Autodesk Inventor part; units mm, degrees
ref_plane "YZ Plane" through (0, 0, 0) normal (1, 0, 0) x (0, 1, 0)
ref_plane "XZ Plane" through (0, 0, 0) normal (0, 1, 0) x (-1, 0, 0)
ref_plane "XY Plane" through (0, 0, 0) normal (0, 0, 1) x (1, 0, 0)
sketch "Sketch1" plane through (0, 0, 0) normal (0, 1, 0) x (-1, 0, 0)
  point P0 (0, 0)
sketch "Sketch2" plane through (0, 0, 0) normal (0, 1, 0) x (-1, 0, 0)
  line L0 (0, 0) -> (35, 0)
  line L1 (35, 0) -> (35, 25)
  line L2 (35, 25) -> (0, 25)
  line L3 (0, 25) -> (0, 0)
  dimension "d0" = 35
  dimension "d1" = 25
extrude "Extrusion1" add sketch "Sketch2" along normal blind 8
sketch "Sketch3" plane through (0, 8, 0) normal (0, 1, 0) x (1, 0, 0)
  line L0 (-28.1608, -22.5) -> (-6.6608, -22.5)
  line L1 (-6.6608, -22.5) -> (-6.6608, -6)
  line L2 (-6.6608, -6) -> (-28.1608, -6)
  line L3 (-28.1608, -6) -> (-28.1608, -22.5)
  dimension "d4" = 21.5
  dimension "d5" = 16.5
extrude "Extrusion2" cut sketch "Sketch3" against normal blind 4
sketch "Sketch4" plane through (-6.6608, 8, 22.5) normal (0, 0, -1) x (-1, 0, 0)
  point P0 (-6.6608, -8)
sketch "Sketch5" plane through (-28.1608, 8, 6) normal (0, 0, 1) x (1, 0, 0)
  line L0 (0, -4) -> (21.5, -4)
  line L1 (21.5, -4) -> (21.5, 0)
  line L2 (21.5, 0) -> (0, 0)
  line L3 (0, 0) -> (0, -4)
  point P0 (28.1608, -8)
sketch "Sketch12" plane through (0, 8, 0) normal (0, 1, 0) x (1, 0, 0)
  line L0 (-28.1608, -6) -> (-6.6608, -6)
  line L1 (0, 0) -> (-35, 0)
  line L2 (-15, -6) -> (-20, -6)
  line L3 (-20, -6) -> (-20, 0)
  line L4 (-20, 0) -> (-15, 0)
  line L5 (-15, 0) -> (-15, -6)
  dimension "d27" = 5
extrude "Extrusion9" cut sketch "Sketch12" against normal blind 2.5
fillet "Fillet1" radius 2 1 edges at (-35, 4, 0)
fillet "Fillet2" radius 2 1 edges at (0, 4, 0)
fillet "Fillet3" radius 2 1 edges at (-35, 4, 25)
fillet "Fillet4" radius 2 1 edges at (0, 4, 25)
fillet "Fillet5" radius 0.5 1 edges at (-17.5, 5.5, 6)
sketch "Sketch13" plane through (0, 0, 0) normal (0, -1, 0) x (1, 0, 0)
  point P0 (0, 0)
sketch "Skizze18" plane through (0, 8, 0) normal (0, 1, 0) x (1, 0, 0)
  circle A0 centre (-3.5, -22.5) radius 1.75
  circle A1 centre (-3.5, -2.5) radius 1.75
  point P0 (0, 0)
  dimension "d47" = 3.5
  dimension "d48" = 3.5
extrude "Extrusion14" cut sketch "Skizze18" against normal blind 20 contours A0
extrude "Extrusion15" cut sketch "Skizze18" against normal blind 20 contours A1
sketch "Skizze19" plane through (0, 8, 0) normal (0, 1, 0) x (1, 0, 0)
  circle A0 centre (-31.5, -22.5) radius 1.75
  point P0 (0, 0)
  dimension "d53" = 3.5
extrude "Extrusion16" cut sketch "Skizze19" against normal blind 20
sketch "Skizze20" plane through (0, 8, 0) normal (0, 1, 0) x (1, 0, 0)
  circle A0 centre (-31.5, -2.5) radius 1.75
  point P0 (0, 0)
  dimension "d56" = 3.5
extrude "Extrusion17" cut sketch "Skizze20" against normal blind 20
sketch "Skizze21" plane through (0, 4, 0) normal (0, 1, 0) x (1, 0, 0)
  circle A0 centre (-10, -19) radius 1.5
  circle A1 centre (-10, -19) radius 1.35
  point P0 (0, 0)
  dimension "d59" = 2.7
extrude "Extrusion18" add sketch "Skizze21" along normal blind 3 contours A1
sketch "Skizze22" plane through (0, 4, 0) normal (0, 1, 0) x (1, 0, 0)
  circle A0 centre (-25, -19) radius 1.5
  circle A1 centre (-25, -19) radius 1.35
  point P0 (0, 0)
  dimension "d62" = 2.7
extrude "Extrusion19" add sketch "Skizze22" along normal blind 2.7 contours A1
fillet "Rundung6" radius 1 1 edges at (-17.5, 5.5, 0)
properties part number "MPU6050_CASE_BOTTOM"
Work out the finished part from the listing and answer in its coordinate system (mm). A direction names the side the tool comes from. Round coordinates to 2 decimals unless told otherwise and drop trailing zeros. Loops run counter-clockwise (first coordinate to the right, second up) from the corner with the lowest first, then second, coordinate; pieces in that order, holes last. Notation, with made-up numbers: M -36.5,-13.5 L -12.5,-13.5 A26 cw -12.5,11.5 Z; hole C -20,2.5 d2. An arc over 180 degrees is marked long. Use CSV: the item, a comma, the result in double quotes.
Q1. A tool of negligible diameter and unlimited length cuts with its end or side. For faces 1 (the flat face through (-17, 4, 0)), 2 (the cylindrical face through (-9.38, 5.48, 17.8)), from which of +Z, -Z, +X, -X, +Y, -Y can it reach the whole face along a straight path? Write none if from no direction.
Determined:
face 1,"-Z, +X, -X, +Y, -Y"
face 2,"+Y"
Q2. Section A-A, the plane z = 2.5 is taken. Determine the outline of the cut face in (x, y), then the cut area to 4 significant figures.
Determined:
outline,"M -35,0 L -33.25,0 L -33.25,8 L -35,8 Z; M -29.75,0 L -5.25,0 L -5.25,8 L -15,8 L -15,5.5 L -20,5.5 L -20,8 L -29.75,8 Z; M -1.75,0 L 0,0 L 0,8 L -1.75,8 Z"
area,"211.5 mm2"
Q3. Each of these flat-tipped pins is pushed along its axis until it touches: pin 1 (3 mm diameter, centred on x = -25.5, z = 19.5, fed in from +Y); pin 2 (2 mm diameter, centred on x = -12, z = 11, fed in from +Y); pin 3 (1.3 mm diameter, centred on x = -10, z = 18.5, fed in from +Y). Where does it stop, or does it pass through?
Determined:
pin 1,"y = 6.7"
pin 2,"y = 4"
pin 3,"y = 7"
Q4. The mould has two halves that part along X. Classify faces 3 (the cylindrical face through (-0.57, 4.06, 0.6)), 4 (the flat face through (-35, 4, 12)), 5 (the flat face through (-10, 7, 19)): pulls with the +X half, pulls with the -X half, needs draft (parallel to the pull), parting line crosses it, or undercut.
Determined:
face 3,"pulls with the +X half"
face 4,"pulls with the -X half"
face 5,"undercut"
Q5. Section B-B, the plane x = -3.5 is taken. Determine the outline of the cut face in (y, z), then the cut area to 3 significant figures.
Determined:
outline,"M 0,0 L 8,0 L 8,0.75 L 0,0.75 Z; M 0,4.25 L 8,4.25 L 8,20.75 L 0,20.75 Z; M 0,24.25 L 8,24.25 L 8,25 L 0,25 Z"
area,"144 mm2"
Q6. Section C-C, the plane y = 2 is taken. Determine the outline of the cut face in (x, z).
Determined:
outline,"M -35,2 A2 ccw -33,0 L -2,0 A2 ccw 0,2 L 0,23 A2 ccw -2,25 L -33,25 A2 ccw -35,23 Z; hole C -31.5,2.5 d3.5; hole C -31.5,22.5 d3.5; hole C -3.5,2.5 d3.5; hole C -3.5,22.5 d3.5"
Q7. Consider L1, parallel to X at y = 3.75, z = 22.5; L2, parallel to Z at x = -3.5, y = 7.75; L3, parallel to Z at x = -22, y = 6.25. Determine where each line is inside the solid, lowest interval first.
Determined:
L1,"-35 to -33.25, -29.75 to -5.25, -1.75 to 0"
L2,"0 to 0.75, 4.25 to 20.75, 24.25 to 25"
L3,"0 to 6, 22.5 to 25"
Q8. Section D-D, the plane x = -17.5 is taken. Determine the outline of the cut face in (y, z), then the cut area to 3 significant figures.
Determined:
outline,"M 0,0 L 4.5,0 A1 ccw 5.5,1 L 5.5,5.5 A0.5 ccw 5,6 L 4,6 L 4,22.5 L 8,22.5 L 8,25 L 0,25 Z"
area,"119 mm2"
